from build123d import *

# Parameters (mm, degrees)
SKETCH5_R           = 38.5
BOSS_EXTRUDE2_DEPTH = 6.36
SKETCH8_R           = 11
CUT_EXTRUDE4_DEPTH  = 55.817420589
BOSS_EXTRUDE3_START = -6.36
SKETCH9_R           = 38.5
BOSS_EXTRUDE3_DEPTH = 6.36
SKETCH10_R          = 3.175
CUT_EXTRUDE5_DEPTH  = 109.197502744
SKETCH12_R          = 3.625
CUT_EXTRUDE6_DEPTH  = 109.197502744
FILLET1_R           = 10


with BuildPart() as part:
    # Sketch5 → Boss-Extrude2 (new body)
    with BuildSketch(Plane(origin=(0, 0, 0), x_dir=(1, 0, 0), z_dir=(0, 1, 0))):
        with Locations(Location((0, 0, 0), (0, 0, 90))):
            Circle(SKETCH5_R)
    extrude(amount=BOSS_EXTRUDE2_DEPTH)

    # Sketch8 → Cut-Extrude4 (cut, through all)
    with BuildSketch(Plane(origin=(0, 6.36, 0), x_dir=(1, 0, 0), z_dir=(0, 1, 0))):
        with Locations(Location((0, 0, 0), (0, 0, 270))):
            Circle(SKETCH8_R)
    extrude(amount=-CUT_EXTRUDE4_DEPTH, mode=Mode.SUBTRACT)

    # Sketch9 → Boss-Extrude3 (add)
    with BuildSketch(Plane(origin=(0, 6.36, 0), x_dir=(1, 0, 0), z_dir=(0, 1, 0)).offset(BOSS_EXTRUDE3_START)):
        with BuildLine():
            Line((-96, 48.5), (96, 48.5))
            Line((96, 48.5), (96, -1.5))
            ThreePointArc((96, -1.5), (0, -49.5), (-96, -1.5))
            Line((-96, -1.5), (-96, 48.5))
        make_face()
        Circle(SKETCH9_R, mode=Mode.SUBTRACT)
    extrude(amount=BOSS_EXTRUDE3_DEPTH)

    # Sketch10 → Cut-Extrude5 (cut, through all)
    with BuildSketch(Plane(origin=(0, 6.36, 0), x_dir=(1, 0, 0), z_dir=(0, 1, 0))):
        with Locations(Location((-76, 28.5, 0), (0, 0, 270))):
            Circle(SKETCH10_R)
        with Locations(Location((-45, -26.5, 0), (0, 0, 270))):
            Circle(SKETCH10_R)
        with Locations(Location((45, -26.5, 0), (0, 0, 90))):
            Circle(SKETCH10_R)
        with Locations(Location((76, 28.5, 0), (0, 0, 90))):
            Circle(SKETCH10_R)
    extrude(amount=-CUT_EXTRUDE5_DEPTH, mode=Mode.SUBTRACT)

    # Sketch12 → Cut-Extrude6 (cut, through all)
    with BuildSketch(Plane(origin=(0, 6.36, 0), x_dir=(1, 0, 0), z_dir=(0, 1, 0))):
        with Locations(Location((1.988059502, 28.430575432, 0), (0, 0, 270))):
            Circle(SKETCH12_R)
        with Locations(Location((23.627570818, -15.936997749, 0), (0, 0, 270))):
            Circle(SKETCH12_R)
        with Locations(Location((-25.61563032, -12.493577683, 0), (0, 0, 270))):
            Circle(SKETCH12_R)
    extrude(amount=-CUT_EXTRUDE6_DEPTH, mode=Mode.SUBTRACT)

    # Fillet1
    fillet1_edges = [part.edges().sort_by_distance(p)[0] for p in [
        (96, 3.18, 1.5),
        (96, 3.18, -48.5),
        (-96, 3.18, -48.5),
        (-96, 3.18, 1.5),
    ]]
    fillet(fillet1_edges, radius=FILLET1_R)


solid = part.part
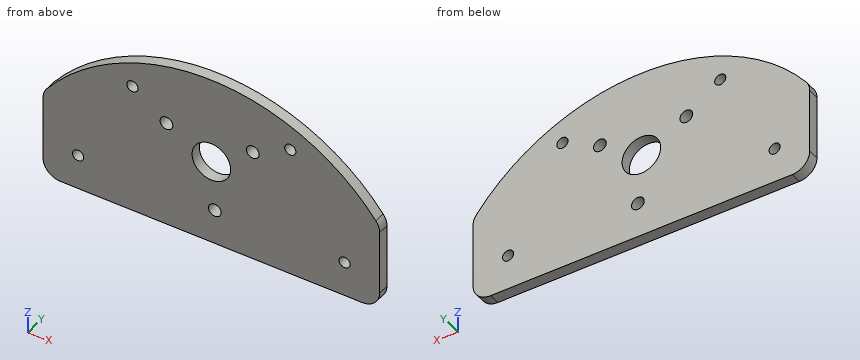
Geometry check sheet. Reference: the model listing, model coordinates, mm. Give positions to 0.01 mm unless a question says otherwise; leave off trailing zeros. Write each loop counter-clockwise with the first axis right and the second up, starting at its lowest first coordinate (ties: lowest second). Pieces come first, ordered by that corner, then holes. Notation, with made-up numbers: M 7,36.25 L 21,36.25 A36 cw 21,73.25 Z; hole C 45.25,67.5 d7. An arc over 180 degrees is marked long. Answer as CSV lines item,"result". Start each with the question number.
Q1. Section check D-D, the plane y = 1.75. Give the number of separate pieces and of enclosed holes in the cut face, then the cut area to 3 significant figures.
Q2. Section check A-A, the plane z = -8. Record the cut outline in (x, y), then the cut area to 3 significant figures.
Q3. Material ranges on L1, parallel to X at y = 2, z = -28.5 (3 decimals); L2, parallel to X at y = 2.25, z = 26.5 (3 decimals); L3, parallel to Z at x = 45, y = 2.5 (3 decimals), recorded low to high.
Q4. Go/stop test with flat-tipped pins: pin 1 (5 mm diameter, centred on x = -45, z = 26.5, fed in from +Y); pin 2 (1.5 mm diameter, centred on y = 1, z = 37, fed in from -X). Record where each tip stops, or that it passes through.
Q5. Section check C-C, the plane z = -28.5. Record the cut outline in (x, y) (3 decimals), then the cut area to 3 significant figures.
Q6. Section check B-B, the plane x = 76. Record the cut outline in (y, z) (1 decimal).
Geometry says:
1,separate pieces,"1"
1,enclosed holes,"8"
1,area,"15,400 mm^2"
2,outline,"M -96,0 L -7.55,0 L -7.55,6.36 L -96,6.36 Z; M 7.55,0 L 96,0 L 96,6.36 L 7.55,6.36 Z"
2,area,"1,130 mm^2"
3,L1,"-96 to -79.175, -72.825 to -1.636, 5.612 to 72.825, 79.175 to 96"
3,L2,"-70.647 to -48.175, -41.825 to 41.825, 48.175 to 70.647"
3,L3,"-48.5 to 23.325, 29.675 to 40.743"
4,pin 1,"through"
4,pin 2,"x = -54.81"
5,outline,"M -96,0 L -79.175,0 L -79.175,6.36 L -96,6.36 Z; M -72.825,0 L -1.636,0 L -1.636,6.36 L -72.825,6.36 Z; M 5.612,0 L 72.825,0 L 72.825,6.36 L 5.612,6.36 Z; M 79.175,0 L 96,0 L 96,6.36 L 79.175,6.36 Z"
5,area,"1,090 mm^2"
6,outline,"M 0,-48.5 L 6.4,-48.5 L 6.4,-31.7 L 0,-31.7 Z; M 0,-25.3 L 6.4,-25.3 L 6.4,22.4 L 0,22.4 Z"
